Autodesk Inventor part; units mm, degrees
ref_plane "YZ Plane" through (0, 0, 0) normal (1, 0, 0) x (0, 1, 0)
ref_plane "XZ Plane" through (0, 0, 0) normal (0, 1, 0) x (-1, 0, 0)
ref_plane "XY Plane" through (0, 0, 0) normal (0, 0, 1) x (1, 0, 0)
sketch "Sketch1" plane through (0, 0, 0) normal (0, 0, 1) x (1, 0, 0)
  line L0 (0, 0) -> (50.8, 0)
  line L1 (50.8, 0) -> (50.8, 95.25)
  line L2 (50.8, 95.25) -> (0, 95.25)
  line L3 (0, 95.25) -> (0, 0)
  dimension "d0" = 50.8
  dimension "d1" = 95.25
extrude "Extrusion1" add sketch "Sketch1" along normal blind 12.7
sketch "Sketch2" plane through (0, 0, 12.7) normal (0, 0, 1) x (1, 0, 0)
  line L0 (0, 0) -> (50.8, 0)
  circle A0 centre (25.4, 74.549) radius 11.303
  dimension "d4" = 74.549
  dimension "d5" = 22.606
extrude "Extrusion2" cut sketch "Sketch2" against normal blind 12.7
properties part number "2f1ah" material "PBT Plastic"
Model file for the job. Use its own axes, mm. Round coordinates to 2 decimals unless told otherwise and drop trailing zeros. Order: outer loops, then holes, each group sorted by start corner. A loop starts at its lowest first (then second) coordinate and runs counter-clockwise, first axis right, second up. Notation, with made-up numbers: (-27, 80.5) -> (11, 80.5) arc R31 ccw to (11, 105.5) -> close; hole circle Ø9 at (29, -38). An arc over 180 degrees is marked (long way). Use one line per item in the form item = value.
Item 1: Cut at A-A, the plane x = 25.4. Write the cut outline in (y, z), and give its area (3 significant figures).
Returned:
outline = (0, 0) -> (63.25, 0) -> (63.25, 12.7) -> (0, 12.7) -> close; (85.85, 0) -> (95.25, 0) -> (95.25, 12.7) -> (85.85, 12.7) -> close
area = 923 mm^2
Item 2: Pull direction Y, two halves, no side cores. Call faces 1 (the face through (26, 95.25, 6)), 2 (the face through (23.929, 85.756, 6.439)), 3 (the face through (25, 0, 6)): released by +Y, released by -Y, zero draft, split by the parting line, or undercut.
Returned:
face_1 = released by +Y
face_2 = undercut
face_3 = released by -Y
Item 3: Drill centre lines: line 1 (Y direction, x = 25.4, z = 3); line 2 (X direction, y = 85, z = 9.5); line 3 (Y direction, x = 22, z = 5). Where is each one in solid material? Low to high.
Returned:
line_1 = 0 to 63.25, 85.85 to 95.25
line_2 = 0 to 21.09, 29.71 to 50.8
line_3 = 0 to 63.77, 85.33 to 95.25
Item 4: Cut at C-C, the plane z = 3.75. Write the cut outline in (x, y).
Returned:
outline = (0, 0) -> (50.8, 0) -> (50.8, 95.25) -> (0, 95.25) -> close; hole circle Ø22.61 at (25.4, 74.55)
Item 5: Cut at B-B, the plane x = 35.5. Write the cut outline in (y, z), and give its area (3 significant figures).
Returned:
outline = (0, 0) -> (69.47, 0) -> (69.47, 12.7) -> (0, 12.7) -> close; (79.62, 0) -> (95.25, 0) -> (95.25, 12.7) -> (79.62, 12.7) -> close
area = 1,080 mm^2
